```python
from build123d import *

# Parameters (mm, degrees)
SKETCH1_W                                           = 132
SKETCH1_H                                           = 20
SKETCH1_R                                           = 1.5
SKETCH1_R_2                                         = 2.5
BOSS_EXTRUDE1_DEPTH                                 = 7
CSK_FOR_M4_COUNTERSUNK_FLAT_HEAD_SCREW1_D           = 3.1
CSK_FOR_M4_COUNTERSUNK_FLAT_HEAD_SCREW1_CSINK_D     = 6
CSK_FOR_M4_COUNTERSUNK_FLAT_HEAD_SCREW1_CSINK_ANGLE = 90


with BuildPart() as part:
    # Sketch1 → Boss-Extrude1 (new body)
    with BuildSketch(Plane.XY):
        Rectangle(SKETCH1_W, SKETCH1_H)
        with Locations((-45, 0)):
            Circle(SKETCH1_R, mode=Mode.SUBTRACT)
        with Locations((45, 0)):
            Circle(SKETCH1_R, mode=Mode.SUBTRACT)
        with Locations((-22, 0)):
            Circle(SKETCH1_R_2, mode=Mode.SUBTRACT)
        with Locations((22, 0)):
            Circle(SKETCH1_R_2, mode=Mode.SUBTRACT)
        with Locations((-58, 0)):
            Circle(SKETCH1_R_2, mode=Mode.SUBTRACT)
        with Locations((58, 0)):
            Circle(SKETCH1_R_2, mode=Mode.SUBTRACT)
    extrude(amount=BOSS_EXTRUDE1_DEPTH)

    # CSK for M4 Countersunk Flat Head Screw1 (through all)
    with Locations(Plane(origin=(-45, 0, 7), x_dir=(1, 0, 0), z_dir=(0, 0, 1))):
        with Locations((0, 0), (90, 0)):
            CounterSinkHole(CSK_FOR_M4_COUNTERSUNK_FLAT_HEAD_SCREW1_D / 2, CSK_FOR_M4_COUNTERSUNK_FLAT_HEAD_SCREW1_CSINK_D / 2, counter_sink_angle=CSK_FOR_M4_COUNTERSUNK_FLAT_HEAD_SCREW1_CSINK_ANGLE)


solid = part.part
```
Model file for the job. Use its own axes, mm. Coordinates: 2 decimals unless noted, no trailing zeros. Order: outer loops, then holes, each group sorted by start corner. A loop starts at its lowest first (then second) coordinate and runs counter-clockwise, first axis right, second up. Notation, with made-up numbers: (-19.5, 66.5) -> (3.5, 66.5) arc R26 cw to (3.5, 95.5) -> close; hole circle Ø8 at (13.5, -23). An arc over 180 degrees is marked (long way). Answer as a JSON object with one key per item and string values. Group by question number.
1) Cut at C-C, the plane x = -45. Write the cut outline in (y, z).
2) Drill centre lines: L1, parallel to Y at x = -58, z = 4; L2, parallel to Y at x = 46, z = 5.5. Where is each one in solid material? Low to high.
3) Flat gauge pins, fed straight in: pin 1 (1.9 mm diameter, centred on x = 45, y = 0, fed in from -Z); pin 2 (5 mm diameter, centred on x = -45, y = 0, fed in from +Z). Where does each tip first touch, or does it go through?
4) Pull direction X, two halves, no side cores. Call faces 1 (the face through (-1, 0, 0)), 2 (the face through (-66, 0, 3)), 3 (the face through (-55.69, -0.96, 3.45)), 4 (the face through (66, 0, 3)): +X half, -X half, draft (parallel to the pull), parting line (faces both ways), or undercut.
5) Cut at A-A, the plane z = 3. Write the cut outline in (x, y), then the cut area to 3 significant figures.
6) Cut at B-B, the plane x = 22. Write the cut outline in (y, z), then the cut area to 3 significant figures.
Check values:
{
 "1": {"outline": "(-10, 0) -> (-1.55, 0) -> (-1.55, 5.55) -> (-3, 7) -> (-10, 7) -> close; (1.55, 0) -> (10, 0) -> (10, 7) -> (3, 7) -> (1.55, 5.55) -> close"},
 "2": {"L1": "y = -10 to -2.5, 2.5 to 10", "L2": "y = -10 to -1.18, 1.18 to 10"},
 "3": {"pin 1": "passes through", "pin 2": "stops at z = 6.5"},
 "4": {"face 1": "draft", "face 2": "-X half", "face 3": "undercut", "face 4": "+X half"},
 "5": {"outline": "(-66, -10) -> (66, -10) -> (66, 10) -> (-66, 10) -> close; hole circle Ø5 at (-58, 0); hole circle Ø3.1 at (-45, 0); hole circle Ø5 at (-22, 0); hole circle Ø5 at (22, 0); hole circle Ø3.1 at (45, 0); hole circle Ø5 at (58, 0)", "area": "2,550 mm²"},
 "6": {"outline": "(-10, 0) -> (-2.5, 0) -> (-2.5, 7) -> (-10, 7) -> close; (2.5, 0) -> (10, 0) -> (10, 7) -> (2.5, 7) -> close", "area": "105 mm²"}
}
